Here's how the part is built. I have some questions about the finished solid (model axes, mm). Give positions to 0.01 mm unless a question says otherwise; leave off trailing zeros. Loops run counter-clockwise (first coordinate to the right, second up) from the corner with the lowest first, then second, coordinate; pieces in that order, holes last. Notation, with made-up numbers: (68.25, 49) - (88.25, 49) arc R19 cw to (88.25, 73) - close; hole circle Ø10 at (35, 15.5). An arc over 180 degrees is marked (long way). One line per item, written item: value. Start each with the question number.
```python
from build123d import *

# Parameters (mm, degrees)
BOSS_EXTRUDE1_DEPTH = 15
SKETCH3_W           = 20
SKETCH3_H           = 10
CUT_EXTRUDE1_DEPTH  = 675
SKETCH4_W           = 20
SKETCH4_H           = 10
CUT_EXTRUDE2_DEPTH  = 751


with BuildPart() as part:
    # Sketch2 → Boss-Extrude1 (new body)
    with BuildSketch(Plane(origin=(0, 0, 0), x_dir=(1, 0, 0), z_dir=(0, 1, 0))):
        Polygon((-375, 300), (-375, -375), (375, -375), (375, 300), (300, 300), (300, 375), (-300, 375), (-300, 300), align=None)
    extrude(amount=BOSS_EXTRUDE1_DEPTH)

    # Sketch3 → Cut-Extrude1 (cut)
    with BuildSketch(Plane.XY.offset(375)):
        with Locations((337.5, 10)):
            Rectangle(SKETCH3_W, SKETCH3_H)
    extrude(amount=-CUT_EXTRUDE1_DEPTH, mode=Mode.SUBTRACT)

    # Sketch4 → Cut-Extrude2 (cut, through all)
    with BuildSketch(Plane(origin=(375, 0, 0), x_dir=(0, 0, -1), z_dir=(1, 0, 0))):
        with Locations((337.5, 10)):
            Rectangle(SKETCH4_W, SKETCH4_H)
    extrude(amount=-CUT_EXTRUDE2_DEPTH, mode=Mode.SUBTRACT)


solid = part.part
```
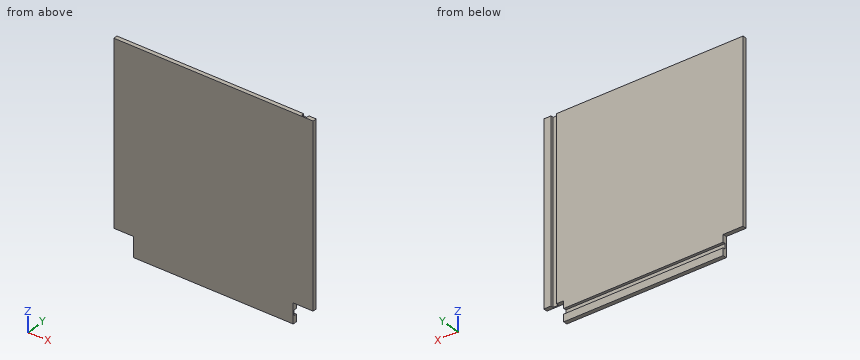
(1) Will these pins go through, and if not, where does the flat tip stop? pin 1 (4.5 mm diameter, centred on y = 6.5, z = -353.5, fed in from +X); pin 2 (4.5 mm diameter, centred on x = 336.5, y = 6, fed in from -Z); pin 3 (6 mm diameter, centred on x = 342, z = 160.5, fed in from +Y).
(2) If we section it at C-C on z = -200: List the corners of the cut face in (x, y) for me.
(3) If we section it at A-A on y = 7.25: List the corners of the cut face in (x, z) for me, plus the area to 3 significant figures.
(4) If we section it at B-B on x = -212: List the corners of the cut face in (y, z) for me, plus the area to 4 significant figures.
(5) Please list where these lines run through material, in increasing order: probe 1 along Z at (x, y) = (205, 9.5); probe 2 along X at (y, z) = (11.25, 103); probe 3 along Y at (x, z) = (340, 263). Write a range as from..to.
Found:
1. pin 1: x = 300
1. pin 2: z = -300
1. pin 3: y = 5
2. outline: (-375, 0) - (375, 0) - (375, 15) - (347.5, 15) - (347.5, 5) - (327.5, 5) - (327.5, 15) - (-375, 15) - close
3. outline: (-375, -300) - (-300, -300) - (-300, -327.5) - (300, -327.5) - (300, -300) - (327.5, -300) - (327.5, 375) - (-375, 375) - close; (-300, -375) - (300, -375) - (300, -347.5) - (-300, -347.5) - close; (347.5, -300) - (375, -300) - (375, 375) - (347.5, 375) - close
3. area: 526,000 mm^2
4. outline: (0, -375) - (15, -375) - (15, -347.5) - (5, -347.5) - (5, -327.5) - (15, -327.5) - (15, 375) - (0, 375) - close
4. area: 11,050 mm^2
5. probe 1: -375..-347.5, -327.5..375
5. probe 2: -375..327.5, 347.5..375
5. probe 3: 0..5
